For this review, take the finished solid that the model builds, in its own axes (mm). Face numbers are marked on the shaded views. A direction names the side the tool comes from. Coordinates: 2 decimals unless noted, no trailing zeros. Write each loop counter-clockwise with the first axis right and the second up, starting at its lowest first coordinate (ties: lowest second). Pieces come first, ordered by that corner, then holes. Notation, with made-up numbers: (81, 87) -> (104, 87) arc R11 cw to (104, 103) -> close; hole circle Ø2 at (26.25, 27). An arc over 180 degrees is marked (long way). Put each result on its own line as item: value. Start each with the question number.
Item 1: Insertion check: P1, Ø6, axis at x = -4.5, y = 1.5, coming from the -Z side; P2, Ø3, axis at x = 4, y = 2.5, coming from the +Z side; P3, Ø8, axis at x = 2, z = 4.5, coming from the -Y side; P4, Ø1.5, axis at y = 3.5, z = 11, coming from the +X side. Each pin has a flat end and moves straight along its axis. Give the tip position at first contact, or say it passes through.
Item 2: Consider section D-D on x = 2. Give the boundary of the cut face in (y, z), and give its area (3 significant figures).
Item 3: To check wall thickness, follow L1, parallel to Z at x = -4, y = 4.75; L2, parallel to Y at x = -13.5, z = 2.75; L3, parallel to X at y = 4.5, z = 1.5. State the ranges of each line that lie inside material, in increasing order.
Item 4: The part is to be moulded in two halves that separate along X. For the marked faces 1 and 2, say which applies: +X half, -X half, draft (parallel to the pull), parting line (faces both ways), or undercut.
Item 5: Consider section A-A on x = -13. Give the boundary of the cut face in (y, z).
Item 6: Consider section C-C on x = 14. Give the boundary of the cut face in (y, z), and give its area (3 significant figures).
Item 7: Consider section B-B on z = 8.25. Give the boundary of the cut face in (x, y).
Item 8: For the marked faces 3 and 4, list the 3-axis set-ups (+Z, -Z, +X, -X, +Y, -Y) from which the entire face can be reached by the end or side of a thin tool; tool diameter is ignored.
```python
from build123d import *

# Parameters (mm, degrees)
F0_W     = 30
F0_H     = 10
F0_R     = 1
F0_R_2   = 0.75
F0_R_3   = 1.25
F0_R_4   = 0.5
F1_DEPTH = 0.25
F2_DEPTH = 15


with BuildPart() as f1:
    # F0 (on Top) → F1 (new body)
    with BuildSketch(Plane.XY):
        with Locations((0, 0.427538)):
            Rectangle(F0_W, F0_H)
        with Locations((-13, -2.572462)):
            Circle(F0_R, mode=Mode.SUBTRACT)
        with Locations((14, -3.572462)):
            Circle(F0_R_2, mode=Mode.SUBTRACT)
        with Locations((-13, 3.427538)):
            Circle(F0_R_3, mode=Mode.SUBTRACT)
        with Locations((14, 4.427538)):
            Circle(F0_R_4, mode=Mode.SUBTRACT)
    extrude(amount=F1_DEPTH)

    # F0 (on Top) → F2 (join)
    with BuildSketch(Plane.XY):
        with Locations((-13, 3.427538)):
            Circle(F0_R_3)
        with Locations((-13, -2.572462)):
            Circle(F0_R)
        with Locations((14, -3.572462)):
            Circle(F0_R_2)
        with Locations((14, 4.427538)):
            Circle(F0_R_4)
    extrude(amount=F2_DEPTH)


solid = f1.part
```
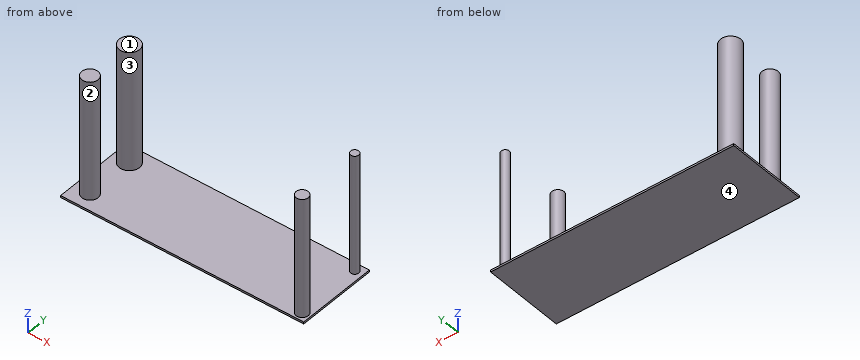
Return value:
1. P1: z = 0
1. P2: z = 0.25
1. P3: through
1. P4: x = 14.47
2. outline: (-4.57, 0) -> (5.43, 0) -> (5.43, 0.25) -> (-4.57, 0.25) -> close
2. area: 2.50 mm^2
3. L1: 0 to 0.25
3. L2: -3.44 to -1.71, 2.28 to 4.57
3. L3: -13.64 to -12.36, 13.51 to 14.49
4. face 1: draft
4. face 2: undercut
5. outline: (-4.57, 0) -> (5.43, 0) -> (5.43, 0.25) -> (4.68, 0.25) -> (4.68, 15) -> (2.18, 15) -> (2.18, 0.25) -> (-1.57, 0.25) -> (-1.57, 15) -> (-3.57, 15) -> (-3.57, 0.25) -> (-4.57, 0.25) -> close
6. outline: (-4.57, 0) -> (5.43, 0) -> (5.43, 0.25) -> (4.93, 0.25) -> (4.93, 15) -> (3.93, 15) -> (3.93, 0.25) -> (-2.82, 0.25) -> (-2.82, 15) -> (-4.32, 15) -> (-4.32, 0.25) -> (-4.57, 0.25) -> close
6. area: 39.4 mm^2
7. outline: circle Ø2.5 at (-13, 3.43); circle Ø2 at (-13, -2.57); circle Ø1.5 at (14, -3.57); circle Ø1 at (14, 4.43)
8. face 3: +Z
8. face 4: -Z, +X, -X, +Y, -Y
